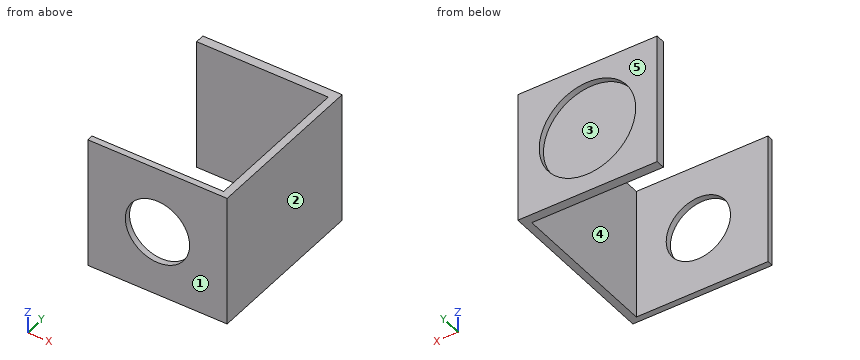
```python
from build123d import *

# Parameters (mm, degrees)
F1_DEPTH = 43
F2_R     = 10.5
F3_DEPTH = 2
F4_R     = 15.75
F5_DEPTH = 2


with BuildPart() as f1:
    # F0 (on Top) → F1 (new body)
    with BuildSketch(Plane.XY):
        Polygon((30.363204, 32.528415), (-15.136796, 32.528415), (-15.136796, 29.528415), (27.863204, 29.528415), (27.863204, -20.471585), (-15.136796, -20.471585), (-15.136796, -22.471585), (30.363204, -22.471585), align=None)
    extrude(amount=F1_DEPTH)

    # F2 (on face) → F3 (cut, through all)
    with BuildSketch(Plane.XZ.offset(22.471585)):
        with Locations((7.613204, 21.5)):
            Circle(F2_R)
    extrude(amount=-F3_DEPTH, mode=Mode.SUBTRACT)

    # F4 (on face) → F5 (cut)
    with BuildSketch(Plane(origin=(0, 32.528415, 0), x_dir=(-1, 0, 0), z_dir=(0, 1, 0))):
        with Locations((-7.613204, 21.5)):
            Circle(F4_R)
    extrude(amount=-F5_DEPTH, mode=Mode.SUBTRACT)


solid = f1.part
```
Geometry: final body of the model. Coordinates: model frame, mm. Face numbers are marked on the shaded views. A direction names the side the tool comes from. Round coordinates to 2 decimals unless told otherwise and drop trailing zeros. Order: outer loops, then holes, each group sorted by start corner. A loop starts at its lowest first (then second) coordinate and runs counter-clockwise, first axis right, second up. Notation, with made-up numbers: M 66.5,-29 L 120.5,-29 A15 cw 120.5,-22 Z; hole C 31,-36.5 d2. An arc over 180 degrees is marked long. One line per item, written item: value.
(1) Cut plane A-A (z = 21.5). Return the cut outline in (x, y).
Result sheet:
outline: M -15.14,-22.47 L -2.89,-22.47 L -2.89,-20.47 L -15.14,-20.47 Z; M -15.14,29.53 L 27.86,29.53 L 27.86,-20.47 L 18.11,-20.47 L 18.11,-22.47 L 30.36,-22.47 L 30.36,32.53 L 23.36,32.53 L 23.36,30.53 L -8.14,30.53 L -8.14,32.53 L -15.14,32.53 Z
(2) Cut plane C-C (x = 22). Return the cut outline in (y, z).
Result sheet:
outline: M -22.47,0 L -20.47,0 L -20.47,43 L -22.47,43 Z; M 29.53,0 L 32.53,0 L 32.53,15.09 L 30.53,15.09 L 30.53,27.91 L 32.53,27.91 L 32.53,43 L 29.53,43 Z
(3) Cut plane D-D (y = -18). Return the cut outline in (x, z), and give its area (4 significant figures).
Result sheet:
outline: M 27.86,0 L 30.36,0 L 30.36,43 L 27.86,43 Z
area: 107.5 mm2
(4) Reachability of the marked faces 4 and 5 from +Z, -Z, +X, -X, +Y, -Y: full face, straight path, thin tool, end or side. Return the list, or none.
Result sheet:
face 4: +Z, -Z, -X
face 5: +Z, -Z, +X, -X, +Y
(5) Cut plane B-B (z = 39). Return the cut outline in (x, y).
Result sheet:
outline: M -15.14,-22.47 L 30.36,-22.47 L 30.36,32.53 L -15.14,32.53 L -15.14,29.53 L 27.86,29.53 L 27.86,-20.47 L -15.14,-20.47 Z
(6) Pin query (flat end, axial travel): P1, Ø3, axis at x = 3, z = 33, coming from the +Y side; P2, Ø8, axis at y = -8, z = 31, coming from the -X side; P3, Ø19, axis at x = 7.61, z = 21.5, coming from the -Y side. Return the tip coordinate at first contact, or that it passes through.
Result sheet:
P1: y = 30.53
P2: x = 27.86
P3: y = 29.53
(7) Line query: probe 1 along Y at (x, z) = (21.5, 35.5); probe 2 along X at (y, z) = (-22, 21); probe 3 along Y at (x, z) = (9, 35.5). Output: solid intervals per line, ascending. Write a range as [from, to].
Result sheet:
probe 1: [-22.47, -20.47], [29.53, 32.53]
probe 2: [-15.14, -2.87], [18.1, 30.36]
probe 3: [-22.47, -20.47], [29.53, 30.53]
(8) Pull-direction query (X, two-part tool) for the marked faces 1, 2 and 3; classes: pulls with the +X half, pulls with the -X half, needs draft (parallel to the pull), parting line crosses it, or undercut.
Result sheet:
face 1: needs draft
face 2: pulls with the +X half
face 3: undercut
